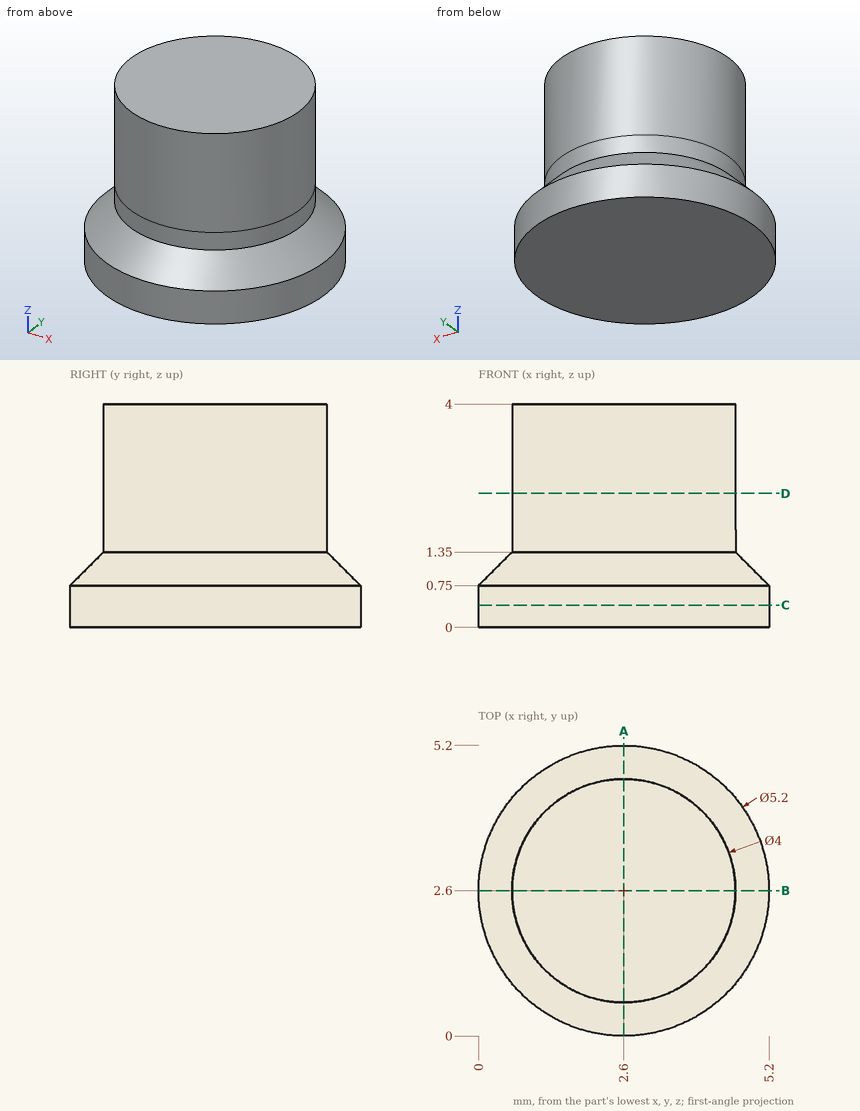
Design review of the part shown in the three views and the two pictorial views. Dimensions are in mm from the part's minimum x, y and z. Round coordinates to 2 decimals unless told otherwise and drop trailing zeros. Loops run counter-clockwise (first coordinate to the right, second up) from the corner with the lowest first, then second, coordinate; pieces in that order, holes last. Notation, with made-up numbers: (84, 6.25) - (119, 6.25) arc R22 ccw to (119, 15.25) - close; hole circle Ø4 at (45, -9). An arc over 180 degrees is marked (long way). Use CSV: the item, a comma, the result in double quotes.
(1) For line 1 (Z direction, x = 0.85, y = 3.75); line 2 (Y direction, x = 3.35, z = 2.6); line 3 (X direction, y = 1, z = 3.3), list the stretches that pass through material, from the lowest coordinate up.
Working result:
line 1,"z = 0 to 1.26"
line 2,"y = 0.75 to 4.45"
line 3,"x = 1.4 to 3.8"
(2) Take a section at C-C, the plane z = 0.4. Give the boundary of the cut face in (x, y), plus the area to 3 significant figures.
Working result:
outline,"circle Ø5.2 at (2.6, 2.6)"
area,"21.2 mm^2"
(3) Clearance check with flat-ended pins moving along their axes: P1, Ø2, axis at x = 1, z = 2.5, coming from the -Y side; P2, Ø1.5, axis at y = 3.5, z = 2, coming from the -X side; P3, Ø1, axis at x = 1.5, y = 2.5, coming from the -Z side; P4, Ø1, axis at x = 4.5, z = 2, coming from the -Y side. State where each tip first meets the part, or that it passes through.
Working result:
P1,"stops at y = 0.69"
P2,"stops at x = 0.61"
P3,"stops at z = 0"
P4,"stops at y = 1.17"
(4) Take a section at A-A, the plane x = 2.6. Give the boundary of the cut face in (y, z).
Working result:
outline,"(0, 0) - (5.2, 0) - (5.2, 0.75) - (4.6, 1.35) - (4.6, 4) - (0.6, 4) - (0.6, 1.35) - (0, 0.75) - close"
(5) Take a section at D-D, the plane z = 2.4. Give the boundary of the cut face in (x, y).
Working result:
outline,"circle Ø4 at (2.6, 2.6)"
